Answer from the drawing. Dimensions are ordinates in mm from the lowest x, y and z of the part. A direction names the side the tool comes from. Round coordinates to 2 decimals unless told otherwise and drop trailing zeros. Order: outer loops, then holes, each group sorted by start corner. A loop starts at its lowest first (then second) coordinate and runs counter-clockwise, first axis right, second up. Notation, with made-up numbers: M 3.5,36 L 22.5,36 A32 ccw 22.5,70 Z; hole C 83,30 d4. An arc over 180 degrees is marked long. Use one line per item in the form item = value. Start each with the question number.
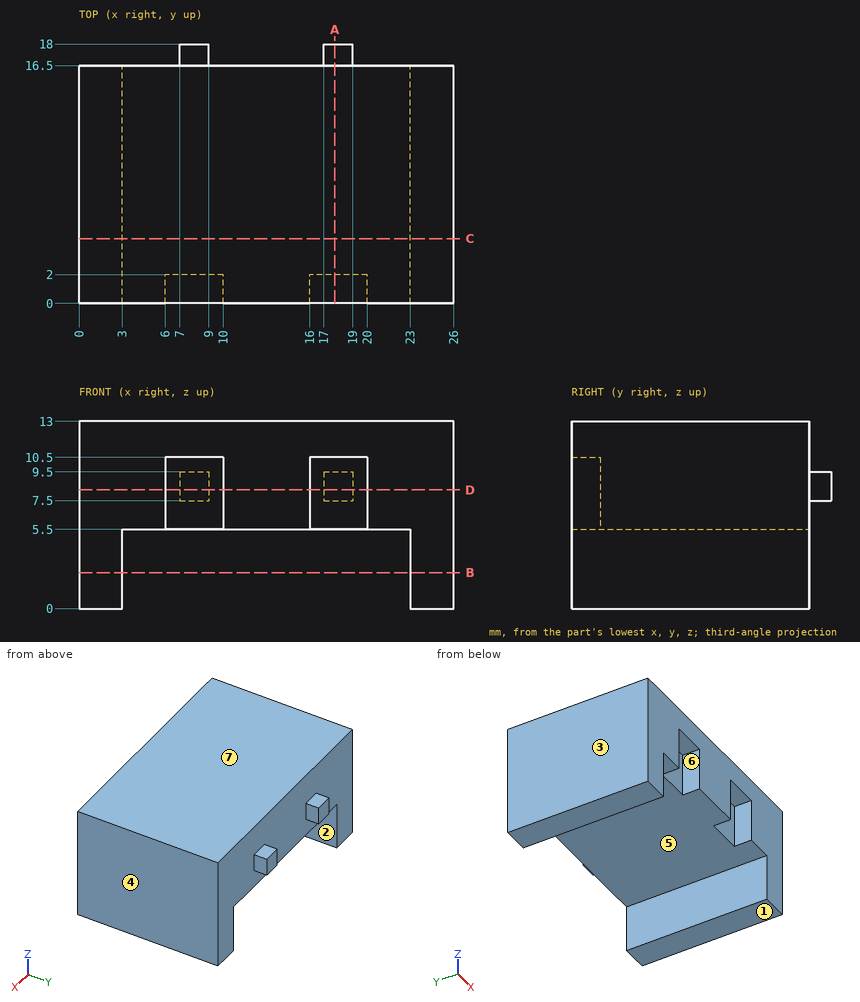
Item 1: A tool of negligible diameter and unlimited length cuts with its end or side. For the marked faces 5, 6 and 7, from which of +Z, -Z, +X, -X, +Y, -Y can it reach the whole face along a straight path? Write none if from no direction.
Item 2: For a pull along X with two mould halves and no side action, classify the marked faces 1, 2, 3 and 4 as pulls with the +X half, pulls with the -X half, needs draft (parallel to the pull), parting line crosses it, or undercut.
Item 3: Section A-A (x = 17.75) is taken. Write down the section's boundary in (y, z).
Item 4: Find the intervals of material crossed by L1, parallel to X at y = 4.75, z = 4.25; L2, parallel to X at y = 1, z = 5.75; L3, parallel to Y at x = 8, z = 6, in increasing order. Write a range as [from, to].
Item 5: Section C-C (y = 4.5) is taken. Write down the section's boundary in (x, z), and give its area (3 significant figures).
Item 6: Section D-D (z = 8.25) is taken. Write down the section's boundary in (x, y), and give its area (3 significant figures).
Item 7: Section B-B (z = 2.5) is taken. Write down the section's boundary in (x, y), and give its area (3 significant figures).
Item 8: Given P1, Ø2, axis at x = 7, z = 5, coming from the +Y side; P2, Ø5, axis at x = 15.5, y = 10, coming from the -Z side; P3, Ø1.6, axis at y = 17, z = 8.5, coming from the -X side; P4, Ø1.2, axis at x = 8.5, y = 17.5, coming from the -Z side, each flat-ended and moving along its own axis, determine where each tip first touches the part or whether it passes through.
The answers:
q1.face_5 = -Z, +Y, -Y
q1.face_6 = -Z, -Y
q1.face_7 = +Z, +X, -X, +Y, -Y
q2.face_1 = needs draft
q2.face_2 = undercut
q2.face_3 = pulls with the -X half
q2.face_4 = pulls with the +X half
q3.outline = M 0,10.5 L 2,10.5 L 2,5.5 L 16.5,5.5 L 16.5,7.5 L 18,7.5 L 18,9.5 L 16.5,9.5 L 16.5,13 L 0,13 Z
q4.L1 = [0, 3], [23, 26]
q4.L2 = [0, 6], [10, 16], [20, 26]
q4.L3 = [2, 16.5]
q5.outline = M 0,0 L 3,0 L 3,5.5 L 23,5.5 L 23,0 L 26,0 L 26,13 L 0,13 Z
q5.area = 228 mm²
q6.outline = M 0,0 L 6,0 L 6,2 L 10,2 L 10,0 L 16,0 L 16,2 L 20,2 L 20,0 L 26,0 L 26,16.5 L 19,16.5 L 19,18 L 17,18 L 17,16.5 L 9,16.5 L 9,18 L 7,18 L 7,16.5 L 0,16.5 Z
q6.area = 419 mm²
q7.outline = M 0,0 L 3,0 L 3,16.5 L 0,16.5 Z; M 23,0 L 26,0 L 26,16.5 L 23,16.5 Z
q7.area = 99.0 mm²
q8.P1 = 16.5
q8.P2 = 5.5
q8.P3 = 0
q8.P4 = 7.5
